```python
from build123d import *

# Parameters (mm, degrees)
F2_R            = 100
F3_DEPTH        = 25
F4_R            = 9
F5_DEPTH        = 1008.001
F5_COPIES_COUNT = 3
F7_DEPTH        = 25


# Not quite as in the source:
# - a pattern or mirror of a feature is missing from the dataset's text; its kind, count and spacing are read off the source's solid


with BuildPart() as f1:
    # F0 (on Right) → F1 (revolve)
    with BuildSketch(Plane.YZ):
        Polygon((12, 600), (0, 600), (0, 0), (8, 0), (8, 544), (1008, 544), (1008, 600), (996, 600), (996, 550), (12, 550), align=None)
    revolve(axis=Axis((0, 4, 0), (0, -1, 0)))

    # F2 (on face) → F3 (cut)
    with BuildSketch(Plane.XZ):
        Circle(F2_R)
    extrude(amount=-F3_DEPTH, mode=Mode.SUBTRACT)

    # F4 (on face) → F5 (cut, through all)
    with BuildSketch(Plane.XZ):
        with Locations((0, 575)):
            Circle(F4_R)
    f5 = extrude(amount=-F5_DEPTH, mode=Mode.SUBTRACT)

    # F5_copies: F5 ×3 about axis
    f5_copies_axis = Axis((0, 0, 0), (0, 1, 0))
    for i in range(1, F5_COPIES_COUNT):
        add(f5.rotate(f5_copies_axis, i * 360 / F5_COPIES_COUNT), mode=Mode.SUBTRACT)

    # F6 (on face) → F7 (cut)
    with BuildSketch(Plane.XZ):
        with BuildLine():
            ThreePointArc((-143.2870199028, 44.3714990436), (-272.593694434, 238.1547264126), (-272, 471.1178196587))
            ThreePointArc((-272, 471.1178196587), (-367.5210729429, 401.0788712247), (-445.6187120932, 312.025581375))
            ThreePointArc((-445.6187120932, 312.025581375), (-362.6540145598, 75.9719974886), (-143.2870199028, -44.3714990436))
            ThreePointArc((-143.2870199028, -44.3714990436), (-150, 0), (-143.2870199028, 44.3714990436))
        make_face()
    extrude(amount=-F7_DEPTH, mode=Mode.SUBTRACT)


solid = f1.part
```
Can you work these out from the model? Positions are in its coordinate system, mm. A direction names the side the tool comes from. Give positions to 0.01 mm unless a question says otherwise; leave off trailing zeros. Order: outer loops, then holes, each group sorted by start corner. A loop starts at its lowest first (then second) coordinate and runs counter-clockwise, first axis right, second up. Notation, with made-up numbers: (18.5, 17.25) - (65.5, 17.25) arc R13 cw to (65.5, 35.25) - close; hole circle Ø2 at (-39.75, -6.75). An arc over 180 degrees is marked (long way). Use a Markdown table: item, result. Add a question column.
Q1. If we section it at A-A on z = -26: Write out the boundary of the cut face in (x, y), plus the area to 3 significant figures.
Q2. If we section it at B-B on x = -213: Write out the boundary of the cut face in (y, z), plus the area to 3 significant figures.
Q3. Please list where these lines run through material, in increasing order: line 1 along Z through (x, y) = (0, 1003.25); line 2 along X through (y, z) = (547, 0); line 3 along X through (y, z) = (998, -287).
Q4. On a 3-axis mill with a long thin cutter (end or side, diameter ignored), from which of +Z, -Z, +X, -X, +Y, -Y can I reach the whole of each face in a straight line? I mean faces 1 (the flat face through (131, 996, -536)), 2 (the flat face through (113, 8, 8)), 3 (the flat face through (125, 0, -8)). Say none if no direction works.
Q5. If we mould it in two halves opening along X, with no side actions, what happens to faces 4 (the cylindrical face through (-594.894, 1001.916, -78.108)), 5 (the cylindrical face through (-364.96, 3.94, 78.72)), 6 (the flat face through (531, 1008, -131))? For each: released by +X, released by -X, zero draft, split by the parting line, or undercut.
Q6. If we section it at C-C on y = 268: Write out the boundary of the cut face in (x, z), plus the area to 3 significant figures.
Q7. I'm going to push flat-ended pins straight in: pin 1 (20.5 mm diameter, centred on x = 0, z = 575, fed in from +Y); pin 2 (2 mm diameter, centred on x = -62, y = 354.5, fed in from +Z); pin 3 (1.5 mm diameter, centred on y = 776.5, z = -219.5, fed in from +X); pin 4 (3 mm diameter, centred on y = 657, z = 45, fed in from -X). Where does each tip first touch, or does it pass through?
Q8. If we section it at D-D on z = 153: Write out the boundary of the cut face in (x, y).
Answers follow:
| question | item | result |
|---|---|---|
| 1 | outline | (-599.44, 0) - (-216.84, 0) - (-216.84, 8) - (-543.38, 8) - (-543.38, 1008) - (-599.44, 1008) - (-599.44, 996) - (-549.39, 996) - (-549.39, 12) - (-599.44, 12) - close; (-147.73, 0) - (-96.56, 0) - (-96.56, 8) - (-147.73, 8) - close; (96.56, 0) - (599.44, 0) - (599.44, 12) - (549.39, 12) - (549.39, 996) - (599.44, 996) - (599.44, 1008) - (543.38, 1008) - (543.38, 8) - (96.56, 8) - close |
| 1 | area | 21,100 mm^2 |
| 2 | outline | (0, -560.92) - (12, -560.92) - (12, -507.08) - (996, -507.08) - (996, -560.92) - (1008, -560.92) - (1008, -500.57) - (8, -500.57) - (8, -27.39) - (0, -27.39) - close; (0, 118.22) - (8, 118.22) - (8, 500.57) - (1008, 500.57) - (1008, 560.92) - (996, 560.92) - (996, 507.08) - (12, 507.08) - (12, 560.92) - (0, 560.92) - close |
| 2 | area | 22,600 mm^2 |
| 3 | line 1 | z = -600 to -544, 544 to 566, 584 to 600 |
| 3 | line 2 | x = -550 to -544, 544 to 550 |
| 3 | line 3 | x = -526.91 to -506.95, -488.98 to -462.13, 462.13 to 488.98, 506.95 to 526.91 |
| 4 | face 1 | none |
| 4 | face 2 | +Y |
| 4 | face 3 | +Z, -Z, +X, -X, -Y |
| 5 | face 4 | split by the parting line |
| 5 | face 5 | undercut |
| 5 | face 6 | zero draft |
| 6 | outline | circle Ø1100 at (0, 0); hole circle Ø1088 at (0, 0) |
| 6 | area | 20,600 mm^2 |
| 7 | pin 1 | stops at y = 1008 |
| 7 | pin 2 | stops at z = 546.61 |
| 7 | pin 3 | stops at x = 504.63 |
| 7 | pin 4 | stops at x = -548.28 |
| 8 | outline | (-580.16, 0) - (-412.27, 0) - (-412.27, 8) - (-522.04, 8) - (-522.04, 1008) - (-580.16, 1008) - (-580.16, 996) - (-528.29, 996) - (-528.29, 12) - (-580.16, 12) - close; (-235.66, 0) - (580.16, 0) - (580.16, 12) - (528.29, 12) - (528.29, 996) - (580.16, 996) - (580.16, 1008) - (522.04, 1008) - (522.04, 8) - (-235.66, 8) - close |
